Verification items for the finished model (mm, model axes). Round coordinates to 2 decimals unless told otherwise and drop trailing zeros. Write each loop counter-clockwise with the first axis right and the second up, starting at its lowest first coordinate (ties: lowest second). Pieces come first, ordered by that corner, then holes. Notation, with made-up numbers: (68.5, 66) - (74.5, 66) arc R25 cw to (74.5, 84) - close; hole circle Ø10 at (77, 41.5). An arc over 180 degrees is marked (long way). Answer as a JSON object with one key per item and string values.
```python
from build123d import *

# Parameters (mm, degrees)
SKETCH_1_R      = 13.1
SKETCH_1_R_2    = 1.6
SKETCH_1_R_3    = 2.1
EXTRUDE_1_DEPTH = 3
FILLET_1_R      = 5


with BuildPart() as part:
    # 草图1 → 凸台-拉伸1 (new body)
    with BuildSketch(Plane.XY):
        with BuildLine():
            Line((-35, 0), (-35, -60))
            Line((-35, -60), (-20, -60))
            Line((-20, -60), (20, -60))
            Line((20, -60), (35, -60))
            Line((35, -60), (35, 0))
            Line((35, 0), (25, 25))
            ThreePointArc((25, 25), (0, 50), (-25, 25))
            Line((-25, 25), (-35, 0))
        make_face()
        with Locations((0, 25)):
            Circle(SKETCH_1_R, mode=Mode.SUBTRACT)
        with Locations((-28, -53)):
            Circle(SKETCH_1_R_2, mode=Mode.SUBTRACT)
        with Locations((-28, -27)):
            Circle(SKETCH_1_R_2, mode=Mode.SUBTRACT)
        with Locations((28, -27)):
            Circle(SKETCH_1_R_2, mode=Mode.SUBTRACT)
        with Locations((28, -53)):
            Circle(SKETCH_1_R_2, mode=Mode.SUBTRACT)
        with Locations((0, 7.5)):
            Circle(SKETCH_1_R_3, mode=Mode.SUBTRACT)
        with Locations((-8.75, 9.844555434)):
            Circle(SKETCH_1_R_3, mode=Mode.SUBTRACT)
        with Locations((-15.155444566, 16.25)):
            Circle(SKETCH_1_R_3, mode=Mode.SUBTRACT)
        with Locations((-17.5, 25)):
            Circle(SKETCH_1_R_3, mode=Mode.SUBTRACT)
        with Locations((-15.155444566, 33.75)):
            Circle(SKETCH_1_R_3, mode=Mode.SUBTRACT)
        with Locations((-8.75, 40.155444566)):
            Circle(SKETCH_1_R_3, mode=Mode.SUBTRACT)
        with Locations((0, 42.5)):
            Circle(SKETCH_1_R_3, mode=Mode.SUBTRACT)
        with Locations((8.75, 40.155444566)):
            Circle(SKETCH_1_R_3, mode=Mode.SUBTRACT)
        with Locations((15.155444566, 33.75)):
            Circle(SKETCH_1_R_3, mode=Mode.SUBTRACT)
        with Locations((17.5, 25)):
            Circle(SKETCH_1_R_3, mode=Mode.SUBTRACT)
        with Locations((15.155444566, 16.25)):
            Circle(SKETCH_1_R_3, mode=Mode.SUBTRACT)
        with Locations((8.75, 9.844555434)):
            Circle(SKETCH_1_R_3, mode=Mode.SUBTRACT)
        with Locations((-3.75, -5)):
            Circle(SKETCH_1_R_2, mode=Mode.SUBTRACT)
        with Locations((3.75, -5)):
            Circle(SKETCH_1_R_2, mode=Mode.SUBTRACT)
        with Locations((3.75, -15)):
            Circle(SKETCH_1_R_2, mode=Mode.SUBTRACT)
        with Locations((-3.75, -15)):
            Circle(SKETCH_1_R_2, mode=Mode.SUBTRACT)
        Polygon((-24.968911087, -38.25), (-28, -36.5), (-31.031088913, -38.25), (-31.031088913, -41.75), (-28, -43.5), (-24.968911087, -41.75), align=None, mode=Mode.SUBTRACT)
        Polygon((-16.968911087, -38.25), (-20, -36.5), (-23.031088913, -38.25), (-23.031088913, -41.75), (-20, -43.5), (-16.968911087, -41.75), align=None, mode=Mode.SUBTRACT)
        Polygon((-8.968911087, -38.25), (-12, -36.5), (-15.031088913, -38.25), (-15.031088913, -41.75), (-12, -43.5), (-8.968911087, -41.75), align=None, mode=Mode.SUBTRACT)
        Polygon((-0.968911087, -38.25), (-4, -36.5), (-7.031088913, -38.25), (-7.031088913, -41.75), (-4, -43.5), (-0.968911087, -41.75), align=None, mode=Mode.SUBTRACT)
        Polygon((7.031088913, -38.25), (4, -36.5), (0.968911087, -38.25), (0.968911087, -41.75), (4, -43.5), (7.031088913, -41.75), align=None, mode=Mode.SUBTRACT)
        Polygon((15.031088913, -38.25), (12, -36.5), (8.968911087, -38.25), (8.968911087, -41.75), (12, -43.5), (15.031088913, -41.75), align=None, mode=Mode.SUBTRACT)
        Polygon((23.031088913, -38.25), (20, -36.5), (16.968911087, -38.25), (16.968911087, -41.75), (20, -43.5), (23.031088913, -41.75), align=None, mode=Mode.SUBTRACT)
        Polygon((31.031088913, -38.25), (28, -36.5), (24.968911087, -38.25), (24.968911087, -41.75), (28, -43.5), (31.031088913, -41.75), align=None, mode=Mode.SUBTRACT)
        Polygon((-16.968911087, -48.25), (-20, -46.5), (-23.031088913, -48.25), (-23.031088913, -51.75), (-20, -53.5), (-16.968911087, -51.75), align=None, mode=Mode.SUBTRACT)
        Polygon((23.031088913, -48.25), (20, -46.5), (16.968911087, -48.25), (16.968911087, -51.75), (20, -53.5), (23.031088913, -51.75), align=None, mode=Mode.SUBTRACT)
        Polygon((-0.968911087, -48.25), (-4, -46.5), (-7.031088913, -48.25), (-7.031088913, -51.75), (-4, -53.5), (-0.968911087, -51.75), align=None, mode=Mode.SUBTRACT)
        Polygon((-8.968911087, -48.25), (-12, -46.5), (-15.031088913, -48.25), (-15.031088913, -51.75), (-12, -53.5), (-8.968911087, -51.75), align=None, mode=Mode.SUBTRACT)
        Polygon((7.031088913, -48.25), (4, -46.5), (0.968911087, -48.25), (0.968911087, -51.75), (4, -53.5), (7.031088913, -51.75), align=None, mode=Mode.SUBTRACT)
        Polygon((15.031088913, -48.25), (12, -46.5), (8.968911087, -48.25), (8.968911087, -51.75), (12, -53.5), (15.031088913, -51.75), align=None, mode=Mode.SUBTRACT)
        Polygon((-16.968911087, -28.25), (-20, -26.5), (-23.031088913, -28.25), (-23.031088913, -31.75), (-20, -33.5), (-16.968911087, -31.75), align=None, mode=Mode.SUBTRACT)
        Polygon((-8.968911087, -28.25), (-12, -26.5), (-15.031088913, -28.25), (-15.031088913, -31.75), (-12, -33.5), (-8.968911087, -31.75), align=None, mode=Mode.SUBTRACT)
        Polygon((-0.968911087, -28.25), (-4, -26.5), (-7.031088913, -28.25), (-7.031088913, -31.75), (-4, -33.5), (-0.968911087, -31.75), align=None, mode=Mode.SUBTRACT)
        Polygon((7.031088913, -28.25), (4, -26.5), (0.968911087, -28.25), (0.968911087, -31.75), (4, -33.5), (7.031088913, -31.75), align=None, mode=Mode.SUBTRACT)
        Polygon((15.031088913, -28.25), (12, -26.5), (8.968911087, -28.25), (8.968911087, -31.75), (12, -33.5), (15.031088913, -31.75), align=None, mode=Mode.SUBTRACT)
        Polygon((23.031088913, -28.25), (20, -26.5), (16.968911087, -28.25), (16.968911087, -31.75), (20, -33.5), (23.031088913, -31.75), align=None, mode=Mode.SUBTRACT)
    extrude(amount=EXTRUDE_1_DEPTH)

    # 圆角1
    fillet_1_edges = [part.edges().sort_by_distance(p)[0] for p in [
        (25, 25, 1.5),
        (35, 0, 1.5),
        (35, -60, 1.5),
        (-35, -60, 1.5),
        (-35, 0, 1.5),
        (-25, 25, 1.5),
    ]]
    fillet(fillet_1_edges, radius=FILLET_1_R)


solid = part.part
```
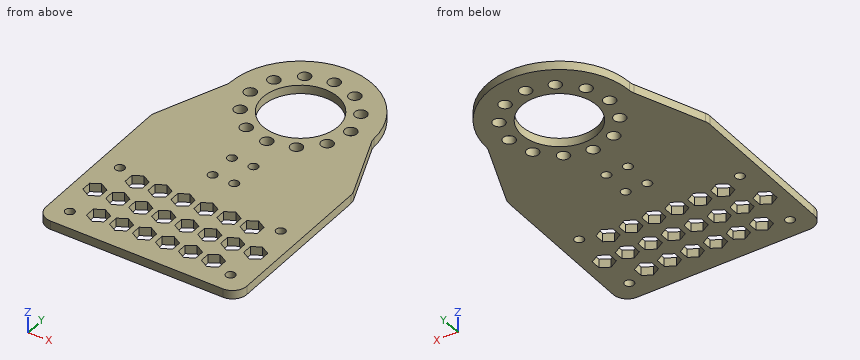
Q1. Section check A-A, the plane y = -5. Record the cut outline in (x, z), then the cut area to 3 significant figures.
Geometry check:
{"outline": "(-35, 0) - (-5.35, 0) - (-5.35, 3) - (-35, 3) - close; (-2.15, 0) - (2.15, 0) - (2.15, 3) - (-2.15, 3) - close; (5.35, 0) - (35, 0) - (35, 3) - (5.35, 3) - close", "area": "191 mm2"}
Q2. Material ranges on line 1 along X through (y, z) = (24.5, 2.35); line 2 along Y through (x, z) = (16, 2.55); line 3 along Y through (x, z) = (21.5, 1.2), recorded low to high. Write a range as [from, to].
Geometry check:
{"line 1": "x = [-25.22, -19.54], [-15.46, -13.09], [13.09, 15.46], [19.54, 25.22]", "line 2": "y = [-60, 14.33], [18.17, 23.53], [26.47, 31.83], [35.67, 44.21]", "line 3": "y = [-60, -52.63], [-47.37, -42.63], [-37.37, -32.63], [-27.37, 37.76]"}
Q3. Gauge pin test, flat end, axial feed: P1, Ø6, axis at x = -6.5, y = -39, coming from the -Z side. Record the tip position at first contact, or that the pin passes through.
Geometry check:
{"P1": "stops at z = 0"}
Q4. Section check B-B, the plane y = 16.25. Record the cut outline in (x, z), then the cut area to 3 significant figures.
Geometry check:
{"outline": "(-28.5, 0) - (-17.26, 0) - (-17.26, 3) - (-28.5, 3) - close; (-13.06, 0) - (-9.75, 0) - (-9.75, 3) - (-13.06, 3) - close; (9.75, 0) - (13.06, 0) - (13.06, 3) - (9.75, 3) - close; (17.26, 0) - (28.5, 0) - (28.5, 3) - (17.26, 3) - close", "area": "87.3 mm2"}
Q5. Section check C-C, the plane z = 1.15. State how many separate pieces and enclosed holes the cut face has, then the cut area to 3 significant figures.
Geometry check:
{"separate pieces": "1", "enclosed holes": "41", "area": "5,260 mm2"}
